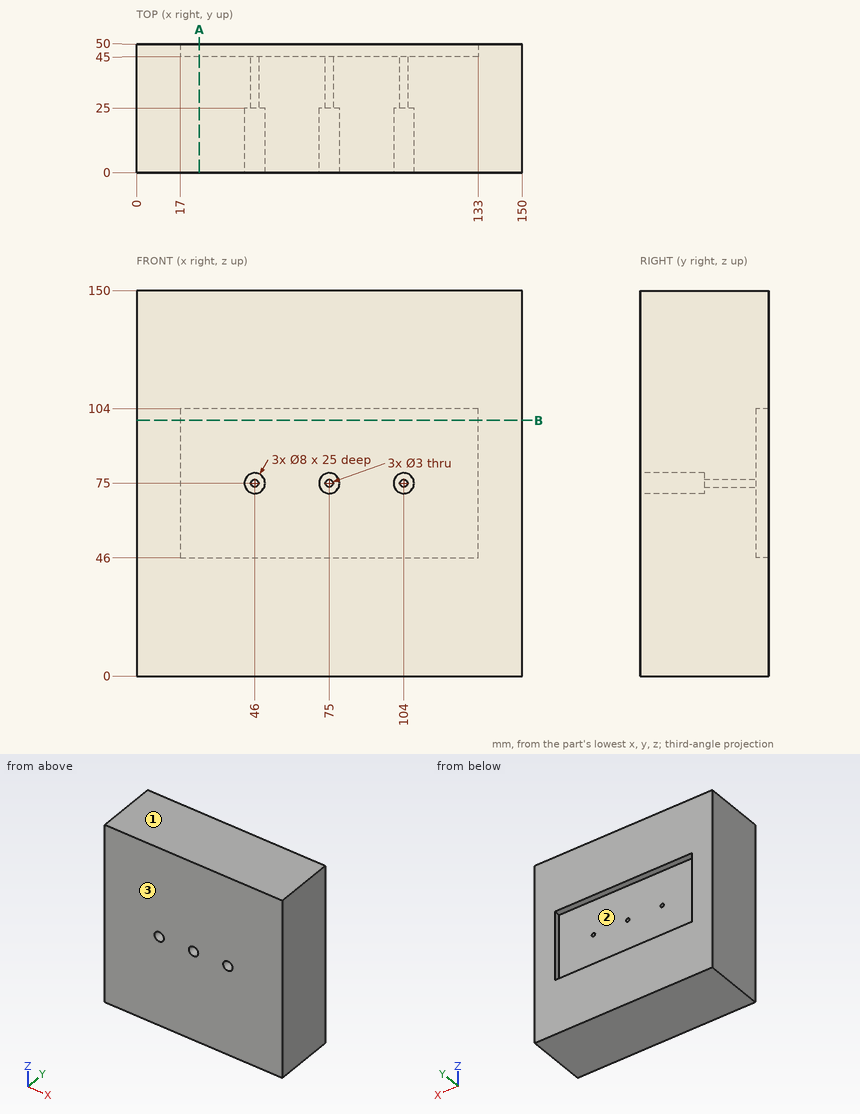
Geometry: see drawing. Coordinates: mm, zero at the bounding-box minimum. Give positions to 0.01 mm unless a question says otherwise; leave off trailing zeros. Write each loop counter-clockwise with the first axis right and the second up, starting at its lowest first coordinate (ties: lowest second). Pieces come first, ordered by that corner, then holes. Notation, with made-up numbers: M 31.5,9.5 L 81.5,9.5 A12 ccw 81.5,22.5 Z; hole C 53.25,-4 d7. An arc over 180 degrees is marked long. Return JSON: item names as keys, results as strings. Group by question number.
1) Ray query, L1, parallel to X at y = 33.5, z = 75; L2, parallel to Z at x = 46, y = 7; L3, parallel to Z at x = 75, y = 39.5. Return the intervals inside material, ascending.
2) First-contact query: pin 1 Ø13 at (x, z) = (75, 75) entering from +Y; pin 2 Ø3.5 at (x, z) = (75, 75) entering from -Y; pin 3 Ø2.5 at (x, z) = (46, 75) entering from +Y. Flat tips, straight axial feed; report the tip coordinate or a pass-through.
3) Draft query along Z for the marked faces 1, 2 and 3. Return one class per face: released by +Z, released by -Z, zero draft, split by the parting line, or undercut.
4) Cut plane A-A, the plane x = 24.5. Output: boundary loops of the cut face in (y, z), then the cut area to 3 significant figures.
5) Cut plane B-B, the plane z = 99.5. Output: boundary loops of the cut face in (x, y), then the cut area to 3 significant figures.
Data:
{
 "1": {"L1": "x = 0 to 44.5, 47.5 to 73.5, 76.5 to 102.5, 105.5 to 150", "L2": "z = 0 to 71, 79 to 150", "L3": "z = 0 to 73.5, 76.5 to 150"},
 "2": {"pin 1": "stops at y = 45", "pin 2": "stops at y = 25", "pin 3": "passes through"},
 "3": {"face 1": "released by +Z", "face 2": "undercut", "face 3": "zero draft"},
 "4": {"outline": "M 0,0 L 50,0 L 50,46 L 45,46 L 45,104 L 50,104 L 50,150 L 0,150 Z", "area": "7,210 mm²"},
 "5": {"outline": "M 0,0 L 150,0 L 150,50 L 133,50 L 133,45 L 17,45 L 17,50 L 0,50 Z", "area": "6,920 mm²"}
}
